```python
from build123d import *
from OCP.BRepFilletAPI import BRepFilletAPI_MakeChamfer

# Parameters (mm, degrees)
BOSS_EXTRUDE1_DEPTH = 3.18
CHAMFER1_SIZE       = 1.59
CHAMFER1_SIZE2      = 10
CHAMFER2_SIZE       = 10
CHAMFER2_SIZE_2     = 1.59
SKETCH2_R           = 41
CUT_EXTRUDE1_DEPTH  = 200


with BuildPart() as part:
    # Sketch1 → Boss-Extrude1 (new body)
    with BuildSketch(Plane.XY):
        Polygon((0, 0), (200, 0), (245, 80.01), (195, 80.01), align=None)
    extrude(amount=BOSS_EXTRUDE1_DEPTH)

    # Chamfer1: one chamfer whose edges measure the first distance from different faces: ONE call of the kernel's chamfer builder (chamfer() names one face for all edges)
    chamfer1_edges_1 = [part.edges().sort_by_distance(p)[0] for p in [
        (222.5, 40.005, 3.18),
    ]]
    chamfer1_side_1 = [part.faces().sort_by_distance(p)[0] for p in [
        (222.5, 40.005, 1.59),
    ]]
    chamfer1_edges_2 = [part.edges().sort_by_distance(p)[0] for p in [
        (220, 80.01, 3.18),
    ]]
    chamfer1_side_2 = [part.faces().sort_by_distance(p)[0] for p in [
        (220, 80.01, 1.59),
    ]]
    chamfer1_edges_3 = [part.edges().sort_by_distance(p)[0] for p in [
        (97.5, 40.005, 3.18),
    ]]
    chamfer1_side_3 = [part.faces().sort_by_distance(p)[0] for p in [
        (97.5, 40.005, 1.59),
    ]]
    chamfer1 = BRepFilletAPI_MakeChamfer(part.part.solid().wrapped)
    for e in chamfer1_edges_1:
        chamfer1.Add(CHAMFER1_SIZE, CHAMFER1_SIZE2, e.wrapped, chamfer1_side_1[0].wrapped)  # the first distance lies on this face
    for e in chamfer1_edges_2:
        chamfer1.Add(CHAMFER1_SIZE, CHAMFER1_SIZE2, e.wrapped, chamfer1_side_2[0].wrapped)  # the first distance lies on this face
    for e in chamfer1_edges_3:
        chamfer1.Add(CHAMFER1_SIZE, CHAMFER1_SIZE2, e.wrapped, chamfer1_side_3[0].wrapped)  # the first distance lies on this face
    add(Compound.cast(chamfer1.Shape()), mode=Mode.REPLACE)

    # Chamfer2
    # the kernel refuses this chamfer: 10, 1.59 mm, written as the material it takes off along each edge
    with BuildSketch(Plane(origin=(187.260266978, -22.651245312, 0), x_dir=(-0.8715858085324353, 0.49020574158179714, -0.006042291378384645), z_dir=(0.4902146903574218, 0.8716017194554959, 0))) as chamfer2_piece_1:
        Polygon((CHAMFER2_SIZE * 0.999981745191, CHAMFER2_SIZE * 0.00604229137838), (-CHAMFER2_SIZE_2 * 0.00604229137837, CHAMFER2_SIZE_2 * 0.999981745191), (0, 0), align=None)
    extrude(amount=143.772651921, mode=Mode.SUBTRACT)
    with BuildSketch(Plane(origin=(219.042912573, 89.874991974, 0), x_dir=(-0.0882418861116751, 0.21506271455788833, 0.9726054690070617), z_dir=(-0.9251519574595215, -0.3795969646991606, 0))) as chamfer2_piece_2:
        Polygon((CHAMFER2_SIZE_2 * 0.972605469007, -CHAMFER2_SIZE_2 * 0.232462043477), (-CHAMFER2_SIZE * 0.232462043477, -CHAMFER2_SIZE * 0.972605469007), (0, 0), align=None)
    extrude(amount=262.752322131, mode=Mode.SUBTRACT)
    with BuildSketch(Plane(origin=(270.98806864, 80.01, 0), x_dir=(0, -0.9999817451908304, -0.006042291378384625), z_dir=(-1, 0, 0))) as chamfer2_piece_3:
        Polygon((CHAMFER2_SIZE * 0.999981745191, CHAMFER2_SIZE * 0.00604229137838), (-CHAMFER2_SIZE_2 * 0.00604229137838, CHAMFER2_SIZE_2 * 0.999981745191), (0, 0), align=None)
    extrude(amount=101.976137281, mode=Mode.SUBTRACT)

    # Sketch2 → Cut-Extrude1 (cut)
    with BuildSketch(Plane(origin=(0, 0, 0), x_dir=(0, 0, -1), z_dir=(1, 0, 0))):
        with Locations((-1.59, -40.969157912)):
            Circle(SKETCH2_R)
    extrude(amount=CUT_EXTRUDE1_DEPTH, mode=Mode.SUBTRACT)


solid = part.part
```
For this review, take the finished solid that the model builds, in its own axes (mm). Give positions to 0.01 mm unless a question says otherwise; leave off trailing zeros. Write each loop counter-clockwise with the first axis right and the second up, starting at its lowest first coordinate (ties: lowest second). Pieces come first, ordered by that corner, then holes. Notation, with made-up numbers: M -12.5,85.25 L 11.5,85.25 A19 ccw 11.5,114.25 Z; hole C 31.25,53 d5. An arc over 180 degrees is marked long. One line per item, written item: value.
1) Take a section at B-B, the plane y = 27.5. Write out the cut boundary in (x, z).
Results are:
outline: M 67.02,1.59 L 93.37,0 L 203.99,0 L 215.47,1.59 L 203.99,3.18 L 93.37,3.18 Z
2) For line 1 (Z direction, x = 51, y = 15.5), list the stretches that pass through material, from the lowest coordinate up. Write a range as from..to.
Results are:
line 1: z = 0.79..2.39
3) Take a section at D-D, the plane y = 10.5. Write out the cut boundary in (x, z).
Results are:
outline: M 25.59,1.59 L 51.93,0 L 194.43,0 L 205.91,1.59 L 194.43,3.18 L 51.93,3.18 Z
4) For P1, Ø1.5, axis at x = 142.5, y = 58.5, coming from the -Z side, flat-tipped, find the tip position at first contact; note if it passes through.
Results are:
P1: stops at z = 1.48
5) Take a section at C-C, the plane z = 1. Write out the cut boundary in (x, y), then the cut area to 3 significant figures.
Results are:
outline: M 9.84,0.03 L 195.76,0.03 L 238.66,76.3 L 195.73,76.3 Z
area: 8,730 mm²
6) Take a section at A-A, the plane x = 170.5. Write out the cut boundary in (y, z), then the cut area to 3 significant figures.
Results are:
outline: M 0,0 L 59.15,0 L 69.96,1.59 L 59.15,3.18 L 0,3.18 A41 cw Z
area: 205 mm²
